Work out the finished part from the listing and answer in its coordinate system (mm). A direction names the side the tool comes from. Coordinates: 2 decimals unless noted, no trailing zeros. Order: outer loops, then holes, each group sorted by start corner. A loop starts at its lowest first (then second) coordinate and runs counter-clockwise, first axis right, second up. Notation, with made-up numbers: M -25.75,62.5 L 4.25,62.5 A26 cw 4.25,83.5 Z; hole C -33,11 d7. An arc over 180 degrees is marked long. Answer in a Markdown table with one row per item. Add a question column.
Item 1: The mould has two halves that part along X. Classify faces 3 (the face through (1.3, -1.3, 9.525)), 4 (the face through (-0.359, -1.616, 6.394)), 5 (the face through (-1.38, -6.2, 5.98)): released by +X, released by -X, zero draft, split by the parting line, or undercut.
Item 2: Which of the six approach directions +Z, -Z, +X, -X, +Y, -Y give full straight-line access (tool end or side, diameter ignored) to faces 1 (the face through (-0.12, -0.56, 1.57)), 2 (the face through (0, -1, 3.175))?
Item 3: The part is cut by section C-C (z = 3.5). Write down the section's boundary in (x, y), then the cut area to 3 significant figures.
Item 4: Flat-ended cylindrical pins translate along their axes: pin 1 Ø5.5 at (x, y) = (0, 0) entering from -Z; pin 2 Ø0.9 at (x, y) = (0, 0) entering from +Z; pin 3 Ø4 at (x, z) = (5, 8) entering from -Y; pin 4 Ø4 at (y, z) = (-3, 4.5) entering from -X. Find the tip coordinate at first contact, or state that the pin passes through.
Item 5: The part is cut by section D-D (z = 2). Write down the section's boundary in (x, y), then the cut area to 3 significant figures.
Item 6: Consider line 1 (Y direction, x = 0, z = 8); line 2 (Y direction, x = 0, z = 1.8); line 3 (X direction, y = 0.75, z = 4.25). Determine where each line is inside the solid, lowest interval first. Write a range as from..to.
from build123d import *

# Parameters (mm, degrees)
F0_R     = 6.35
F0_R_2   = 0.5715
F1_DEPTH = 9.525
F2_R     = 1.655421
F2_R_2   = 0.5715
F3_DEPTH = 6.35
F4_R     = 2.54


with BuildPart() as f1:
    # F0 (on Top) → F1 (new body)
    with BuildSketch(Plane.XY):
        Circle(F0_R)
        Circle(F0_R_2, mode=Mode.SUBTRACT)
    extrude(amount=F1_DEPTH)

    # F2 (on face) → F3 (cut)
    with BuildSketch(Plane.XY.offset(9.525)):
        Circle(F2_R)
        Circle(F2_R_2, mode=Mode.SUBTRACT)
    extrude(amount=-F3_DEPTH, mode=Mode.SUBTRACT)

    # F4
    f4_edges = [f1.edges().sort_by_distance(p)[0] for p in [
        (-6.35, 0, 0),
    ]]
    fillet(f4_edges, radius=F4_R)


solid = f1.part
Reply:
| question | item | result |
|---|---|---|
| 1 | face 3 | zero draft |
| 1 | face 4 | undercut |
| 1 | face 5 | split by the parting line |
| 2 | face 1 | +Z, -Z |
| 2 | face 2 | +Z |
| 3 | outline | C 0,0 d12.7; hole C 0,0 d3.31 |
| 3 | area | 118 mm2 |
| 4 | pin 1 | stops at z = 0 |
| 4 | pin 2 | passes through |
| 4 | pin 3 | stops at y = -5.6 |
| 4 | pin 4 | stops at x = -6.27 |
| 5 | outline | C 0,0 d12.58; hole C 0,0 d1.14 |
| 5 | area | 123 mm2 |
| 6 | line 1 | y = -6.35..-1.66, 1.66..6.35 |
| 6 | line 2 | y = -6.24..-0.57, 0.57..6.24 |
| 6 | line 3 | x = -6.31..-1.48, 1.48..6.31 |
